```python
from build123d import *

# Parameters (mm, degrees)
BOSS_EXTRUDE1_DEPTH          = 19.05
M2_5X0_45_TAPPED_HOLE1_D     = 2.05
SKETCH6_OUTSIDE_W            = 56.088
SKETCH6_OUTSIDE_H            = 68.788
SKETCH6_OUTSIDE_R            = 3
CUT_EXTRUDE1_DEPTH           = 2
CUT_EXTRUDE1_TAPER           = 30
SKETCH7_W                    = 15.875
SKETCH7_H                    = 12.7
CUT_EXTRUDE2_DEPTH           = 3.0000001
CUT_EXTRUDE2_DEPTH_BACK      = 24.4
F_10_0_1935_DIAMETER_HOLE1_D = 4.9149


with BuildPart() as part:
    # Sketch1 → Boss-Extrude1 (new body, symmetric)
    with BuildSketch(Plane(origin=(0, 0, 0), x_dir=(0, 0, -1), z_dir=(1, 0, 0))):
        with BuildLine():
            Line((25.4, 0), (0, 0))
            Line((0, 0), (0, 50.8))
            Line((0, 50.8), (6.35, 50.8))
            Line((6.35, 50.8), (6.35, 12.7))
            ThreePointArc((6.35, 12.7), (8.209871939, 8.209871939), (12.7, 6.35))
            Line((12.7, 6.35), (25.4, 6.35))
            Line((25.4, 6.35), (25.4, 0))
        make_face()
    extrude(amount=BOSS_EXTRUDE1_DEPTH, both=True)

    # M2.5x0.45 Tapped Hole1 (through all)
    with Locations(Plane.XY):
        with Locations((-14, 45.75), (14, 45.75), (14, 17.75), (-14, 17.75)):
            Hole(M2_5X0_45_TAPPED_HOLE1_D / 2)

    # Sketch6 outside → Cut-Extrude1 (cut)
    with BuildSketch(Plane.XY):
        with Locations((0, 25.4)):
            Rectangle(SKETCH6_OUTSIDE_W, SKETCH6_OUTSIDE_H)
        with Locations((-14, 45.75)):
            Circle(SKETCH6_OUTSIDE_R, mode=Mode.SUBTRACT)
        with Locations((14, 45.75)):
            Circle(SKETCH6_OUTSIDE_R, mode=Mode.SUBTRACT)
        with Locations((14, 17.75)):
            Circle(SKETCH6_OUTSIDE_R, mode=Mode.SUBTRACT)
        with Locations((-14, 17.75)):
            Circle(SKETCH6_OUTSIDE_R, mode=Mode.SUBTRACT)
    extrude(amount=-CUT_EXTRUDE1_DEPTH, taper=CUT_EXTRUDE1_TAPER, mode=Mode.SUBTRACT)

    # Sketch7 → Cut-Extrude2 (cut, two sides)
    with BuildSketch(Plane.XY.offset(-2)) as cut_extrude2_sk:
        with Locations((-4.15, 18.225)):
            Rectangle(SKETCH7_W, SKETCH7_H)
    extrude(amount=CUT_EXTRUDE2_DEPTH, mode=Mode.SUBTRACT)
    extrude(cut_extrude2_sk.sketch, amount=-CUT_EXTRUDE2_DEPTH_BACK, mode=Mode.SUBTRACT)

    # #10 (0.1935) Diameter Hole1 (through all)
    with Locations(Plane(origin=(0, 6.35, 0), x_dir=(1, 0, 0), z_dir=(0, 1, 0))):
        with Locations((-12.7, 19.05), (0, 19.05), (12.7, 19.05)):
            Hole(F_10_0_1935_DIAMETER_HOLE1_D / 2)


solid = part.part
```
Input: part model. Units: mm. Frame: model coordinates. A direction names the side the tool comes from. Coordinates: 2 decimals unless noted, no trailing zeros. Loops run counter-clockwise (first coordinate to the right, second up) from the corner with the lowest first, then second, coordinate; pieces in that order, holes last. Notation, with made-up numbers: M 25.25,73 L 63.25,73 A27 ccw 63.25,94 Z; hole C 12,60.25 d8. An arc over 180 degrees is marked long. Answer in a Markdown table with one row per item.
1. Reachability of faces 1 (the flat face through (0, 25, -2)), 2 (the flat face through (-4, 11.875, -4)), 3 (the cylindrical face through (-13.83, 3.13, -16.87)) from +Z, -Z, +X, -X, +Y, -Y: full face, straight path, thin tool, end or side. Return the list, or none.
Response:
| item | result |
|---|---|
| face 1 | +Z |
| face 2 | +Z, -Z |
| face 3 | +Y, -Y |
2. Section A-A, the plane z = -19.05. Output: boundary loops of the cut face in (x, y).
Response:
| item | result |
|---|---|
| outline | M -19.05,0 L -15.16,0 L -15.16,6.35 L -19.05,6.35 Z; M -10.24,0 L -2.46,0 L -2.46,6.35 L -10.24,6.35 Z; M 2.46,0 L 10.24,0 L 10.24,6.35 L 2.46,6.35 Z; M 15.16,0 L 19.05,0 L 19.05,6.35 L 15.16,6.35 Z |
3. First-contact query: pin 1 (3 mm diameter, centred on x = 0, z = -19.05, fed in from +Y); pin 2 (19 mm diameter, centred on x = -3.5, y = 24, fed in from -Z); pin 3 (8 mm diameter, centred on x = 12.7, z = -19.05, fed in from +Y); pin 4 (11.5 mm diameter, centred on x = 6.5, y = 25, fed in from +Z). Flat tips, straight axial feed; report the tip coordinate or a pass-through.
Response:
| item | result |
|---|---|
| pin 1 | passes through |
| pin 2 | stops at z = -6.35 |
| pin 3 | stops at y = 6.35 |
| pin 4 | stops at z = -2 |
4. Material intervals for line 1 (Y direction, x = -14, z = -3) (3 decimals); line 2 (Y direction, x = -14, z = -1.5) (3 decimals); line 3 (Z direction, x = -6, y = 40), sorted ascending.
Response:
| item | result |
|---|---|
| line 1 | y = 0 to 16.725, 18.775 to 44.725, 46.775 to 50.8 |
| line 2 | y = 13.884 to 16.725, 18.775 to 21.616, 41.884 to 44.725, 46.775 to 49.616 |
| line 3 | z = -6.35 to -2 |
5. Section C-C, the plane x = -14. Output: boundary loops of the cut face in (y, z) (3 decimals), then the cut area to 3 significant figures.
Response:
| item | result |
|---|---|
| outline | M 0,-25.4 L 6.35,-25.4 L 6.35,-21.135 L 0,-21.135 Z; M 0,-16.965 L 6.35,-16.965 L 6.35,-12.7 A6.35 cw 12.7,-6.35 L 16.725,-6.35 L 16.725,0 L 14.75,0 L 13.595,-2 L 0,-2 Z; M 18.775,-6.35 L 44.725,-6.35 L 44.725,0 L 42.75,0 L 41.595,-2 L 21.905,-2 L 20.75,0 L 18.775,0 Z; M 46.775,-6.35 L 50.8,-6.35 L 50.8,-2 L 49.905,-2 L 48.75,0 L 46.775,0 Z |
| area | 327 mm2 |
6. Section B-B, the plane y = 24. Output: boundary loops of the cut face in (x, z), then the cut area to 3 significant figures.
Response:
| item | result |
|---|---|
| outline | M -19.05,-6.35 L -12.09,-6.35 L -12.09,-2 L -19.05,-2 Z; M 3.79,-6.35 L 19.05,-6.35 L 19.05,-2 L 3.79,-2 Z |
| area | 96.7 mm2 |
7. Draft query along Y for faces 4 (the flat face through (0, 0, -14)), 5 (the cylindrical face through (14.133, 18.766, -3.219)), 6 (the flat face through (19.05, 16, -6)), 7 (the cylindrical face through (0.27, 8.26, -8.16)). Return one class per face: pulls with the +Y half, pulls with the -Y half, needs draft (parallel to the pull), parting line crosses it, or undercut.
Response:
| item | result |
|---|---|
| face 4 | pulls with the -Y half |
| face 5 | undercut |
| face 6 | needs draft |
| face 7 | pulls with the +Y half |
8. Section D-D, the plane y = 17.75. Count the separate pieces of the cut face and the enclosed holes in it, then the cut area to 3 significant figures.
Response:
| item | result |
|---|---|
| separate pieces | 4 |
| enclosed holes | 0 |
| area | 95.9 mm2 |
